```python
from build123d import *

# Parameters (mm, degrees)
F0_W     = 19.05
F0_H     = 19.05
F1_DEPTH = 106.68
F3_D     = 4.0386
F3_DEPTH = 19.05
F3_TIP   = 1.213317848
F5_D     = 6.9088
F5_DEPTH = 24.3416666667
F5_TIP   = 2.0756129224


with BuildPart() as f1:
    # F0 (on Top) → F1 (new body)
    with BuildSketch(Plane.XY):
        with Locations((9.525, 9.525)):
            Rectangle(F0_W, F0_H)
    extrude(amount=F1_DEPTH)

    # F3
    with Locations(Plane.XY.offset(106.68)):
        with Locations((12.7, 12.7), (6.35, 6.35)):
            Hole(F3_D / 2, depth=F3_DEPTH)
            with Locations((0, 0, -(F3_DEPTH + F3_TIP / 2))):  # 118° drill point
                Cone(0, F3_D / 2, F3_TIP, mode=Mode.SUBTRACT)

    # F5
    with Locations(Plane(origin=(0, 0, 0), x_dir=(1, 0, 0), z_dir=(0, 0, -1))):
        with Locations((9.525, -9.525)):
            Hole(F5_D / 2, depth=F5_DEPTH)
            with Locations((0, 0, -(F5_DEPTH + F5_TIP / 2))):  # 118° drill point
                Cone(0, F5_D / 2, F5_TIP, mode=Mode.SUBTRACT)


solid = f1.part
```
For this review, take the finished solid that the model builds, in its own axes (mm). A direction names the side the tool comes from. Coordinates: 2 decimals unless noted, no trailing zeros. Write each loop counter-clockwise with the first axis right and the second up, starting at its lowest first coordinate (ties: lowest second). Pieces come first, ordered by that corner, then holes. Notation, with made-up numbers: (-2.75, 68) - (10.25, 68) arc R14 ccw to (10.25, 84) - close; hole circle Ø4 at (0, 28). An arc over 180 degrees is marked (long way). Put each result on its own line as item: value.
1. For pin 1 (4 mm diameter, centred on x = 9.525, y = 9.525, fed in from -Z); pin 2 (3.5 mm diameter, centred on x = 6.35, y = 6.35, fed in from +Z), all flat-tipped, find the tip position at first contact; note any pin that passes through.
Values found:
pin 1: z = 25.22
pin 2: z = 87.47
2. Machinability: for faces 1 (the flat face through (9, 0, 53)), 2 (the cylindrical face through (12.976, 9.373, 12.341)), which of the approach directions +Z, -Z, +X, -X, +Y, -Y give a long, thin tool a straight path to every point of the face, cutting with its end or side? Answer none if there is none.
Values found:
face 1: +Z, -Z, +X, -X, -Y
face 2: -Z
3. Add section A-A, the plane z = 93. Give the boundary of the cut face in (x, y).
Values found:
outline: (0, 0) - (19.05, 0) - (19.05, 19.05) - (0, 19.05) - close; hole circle Ø4.04 at (6.35, 6.35); hole circle Ø4.04 at (12.7, 12.7)
4. Wall thickness on probe 1 along Y at (x, z) = (12.7, 93.5); probe 2 along X at (y, z) = (6.35, 99.5): over which ranges is each line inside the solid? List them lowest first.
Values found:
probe 1: 0 to 10.68, 14.72 to 19.05
probe 2: 0 to 4.33, 8.37 to 19.05
5. Mouldability with a two-part tool opening along X and no side actions: class faces 3 (the flat face through (0, 9, 53)), 4 (the cylindrical face through (4.485, 5.577, 97.022)), 5 (the cylindrical face through (14.3, 11.47, 97.02)), 6 (the flat face through (9, 10, 106.68)) as released by +X, released by -X, zero draft, split by the parting line, or undercut.
Values found:
face 3: released by -X
face 4: undercut
face 5: undercut
face 6: zero draft
6. Add section B-B, the plane z = 22. Give the boundary of the cut face in (x, y) (3 decimals), then the cut area to 3 significant figures.
Values found:
outline: (0, 0) - (19.05, 0) - (19.05, 19.05) - (0, 19.05) - close; hole circle Ø6.909 at (9.525, 9.525)
area: 325 mm²
